Design review of the part built by this model. Coordinates are the model's own, in mm. Round coordinates to 2 decimals unless told otherwise and drop trailing zeros. Loops run counter-clockwise (first coordinate to the right, second up) from the corner with the lowest first, then second, coordinate; pieces in that order, holes last. Notation, with made-up numbers: (10, 42.5) -> (46, 42.5) arc R6 ccw to (46, 51.5) -> close; hole circle Ø11 at (88.5, 53). An arc over 180 degrees is marked (long way). Write each question's results on one line, items separated by ' | '. Start each with the question number.
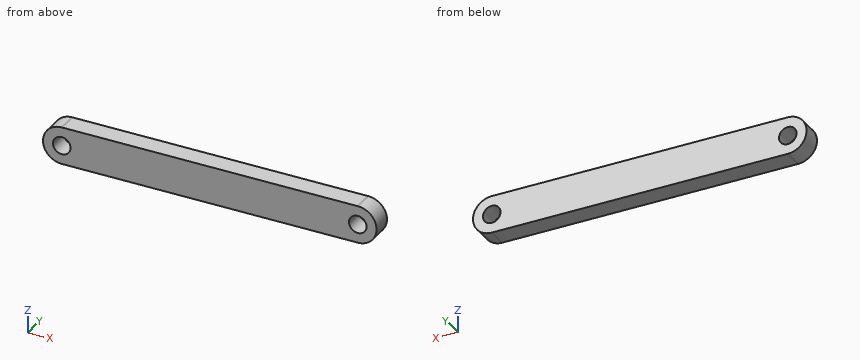
from build123d import *

# Parameters (mm, degrees)
F0_R     = 2.5019
F1_DEPTH = 5.6642


with BuildPart() as f1:
    # F0 (on Front) → F1 (new body)
    with BuildSketch(Plane.XZ):
        with BuildLine():
            ThreePointArc((41.956571, -5.333796), (42.123493, -5.336407), (42.290415, -5.333796))
            Line((42.290415, -5.333796), (41.956571, -5.333796))
        make_face()
        with BuildLine():
            Line((41.956571, -5.333796), (42.290415, -5.333796))
            ThreePointArc((42.290415, -5.333796), (47.4599, 0), (42.290415, 5.333796))
            Line((42.290415, 5.333796), (41.956571, 5.333796))
            Line((41.956571, 5.333796), (-41.956571, 5.333796))
            Line((-41.956571, 5.333796), (-42.290415, 5.333796))
            ThreePointArc((-42.290415, 5.333796), (-47.4599, 0), (-42.290415, -5.333796))
            Line((-42.290415, -5.333796), (-41.956571, -5.333796))
            Line((-41.956571, -5.333796), (41.956571, -5.333796))
        make_face()
        with Locations((-42.123493, 0)):
            Circle(F0_R, mode=Mode.SUBTRACT)
        with Locations((42.123493, 0)):
            Circle(F0_R, mode=Mode.SUBTRACT)
        with BuildLine():
            Line((41.956571, 5.333796), (42.290415, 5.333796))
            ThreePointArc((42.290415, 5.333796), (42.123493, 5.336407), (41.956571, 5.333796))
        make_face()
        with BuildLine():
            ThreePointArc((-42.290415, -5.333796), (-42.123493, -5.336407), (-41.956571, -5.333796))
            Line((-41.956571, -5.333796), (-42.290415, -5.333796))
        make_face()
        with BuildLine():
            Line((-42.290415, 5.333796), (-41.956571, 5.333796))
            ThreePointArc((-41.956571, 5.333796), (-42.123493, 5.336407), (-42.290415, 5.333796))
        make_face()
    extrude(amount=F1_DEPTH)


solid = f1.part
1) Take a section at C-C (z = 4). Write out the cut boundary in (x, y), plus the area to 3 significant figures.
2) Take a section at D-D (z = -3.5). Write out the cut boundary in (x, y), plus the area to 3 significant figures.
3) Take a section at B-B (z = 0). Write out the cut boundary in (x, y).
4) Take a section at A-A (y = -3.5). Write out the cut boundary in (x, z).
5) Insertion check: pin 1 (1.7 mm diameter, centred on x = 4.5, y = -3, fed in from -Z); pin 2 (1.7 mm diameter, centred on x = 15, y = -3, fed in from +Z); pin 3 (5 mm diameter, centred on x = 12.5, z = -3, fed in from +Y); pin 4 (2 mm diameter, centred on y = -1, z = 2.5, fed in from -X). Each pin has a flat end and moves straight along its axis. Give the tip position at first contact, or say it passes through.
6) To check wall thickness, follow line 1 (X direction, y = -2.3, z = 0.5); line 2 (Z direction, x = 37.5, y = -4); line 3 (X direction, y = -3.25, z = -1.25). State the ranges of each line that lie inside material, in increasing order. Write a range as from..to.
Geometry check:
1) outline: (-45.66, -5.66) -> (45.66, -5.66) -> (45.66, 0) -> (-45.66, 0) -> close | area: 517 mm^2
2) outline: (-46.15, -5.66) -> (46.15, -5.66) -> (46.15, 0) -> (-46.15, 0) -> close | area: 523 mm^2
3) outline: (-47.46, -5.66) -> (-44.63, -5.66) -> (-44.63, 0) -> (-47.46, 0) -> close; (-39.62, -5.66) -> (39.62, -5.66) -> (39.62, 0) -> (-39.62, 0) -> close; (44.63, -5.66) -> (47.46, -5.66) -> (47.46, 0) -> (44.63, 0) -> close
4) outline: (-42.29, -5.33) arc R5.34 ccw to (-41.96, -5.33) -> (41.96, -5.33) arc R5.34 ccw to (42.29, -5.33) arc R5.34 ccw to (42.29, 5.33) arc R5.34 ccw to (41.96, 5.33) -> (-41.96, 5.33) arc R5.34 ccw to (-42.29, 5.33) arc R5.34 ccw to start; hole circle Ø5 at (-42.12, 0); hole circle Ø5 at (42.12, 0)
5) pin 1: stops at z = -5.33 | pin 2: stops at z = 5.33 | pin 3: stops at y = 0 | pin 4: stops at x = -47.24
6) line 1: x = -47.44..-44.57, -39.67..39.67, 44.57..47.44 | line 2: z = -5.33..5.33 | line 3: x = -47.31..-44.29, -39.96..39.96, 44.29..47.31
